from build123d import *

# Parameters (mm, degrees)
ESQUISSE1_R             = 16.5
BOSS_EXTRU_1_DEPTH      = 71
ESQUISSE2_R             = 3
BOSS_EXTRU_2_DEPTH      = 20
ESQUISSE3_W             = 2.683906319
ESQUISSE3_H             = 8.065697874
ENL_V_MAT_EXTRU_1_DEPTH = 23


with BuildPart() as part:
    # Esquisse1 → Boss.-Extru.1 (new body)
    with BuildSketch(Plane.XY):
        with Locations((-3.936360625, 11.828431373)):
            Circle(ESQUISSE1_R)
    extrude(amount=BOSS_EXTRU_1_DEPTH)

    # Esquisse2 → Boss.-Extru.2 (add)
    with BuildSketch(Plane.XY.offset(71)):
        with Locations((-3.936360625, 11.828431373)):
            Circle(ESQUISSE2_R)
    extrude(amount=BOSS_EXTRU_2_DEPTH)

    # Esquisse3 → Enlèv. mat.-Extru.1 (cut)
    with BuildSketch(Plane.XY.offset(71)):
        with Locations((-7.643790541, 11.335031517)):
            Rectangle(ESQUISSE3_W, ESQUISSE3_H)
    extrude(amount=ENL_V_MAT_EXTRU_1_DEPTH, mode=Mode.SUBTRACT)


solid = part.part
Build history of the part. All positions in model axes, mm. A direction names the side the tool comes from. Coordinates: 2 decimals unless noted, no trailing zeros. Order: outer loops, then holes, each group sorted by start corner. A loop starts at its lowest first (then second) coordinate and runs counter-clockwise, first axis right, second up. Notation, with made-up numbers: M 83.5,77 L 97.5,77 A24 cw 97.5,112 Z; hole C 6.5,-35 d11. An arc over 180 degrees is marked long. One line per question, with ' | ' between items. Start each with the question number.
Q1. Probe L1, parallel to Z at x = -15, y = 23.5; L2, parallel to Y at x = -4, z = 71.5; L3, parallel to X at y = 12.5, z = 20. List the from-to ranges inside material, lowest first. Write a range as from..to.
Q2. Saw through at D-D (y = 5). List the corners of the cut face in (x, z).
Q3. Saw through at C-C (y = 25). List the corners of the cut face in (x, z).
Q4. 3-axis set-ups, long thin cutter, end or side, ignore diameter. For faces 1 (the face through (-4, 12, 0)), 2 (the face through (-0.94, 11.72, 80.86)), 3 (the face through (-6.302, 12, 81)): which of +Z, -Z, +X, -X, +Y, -Y reach the whole face in a straight line?
Q5. Flat gauge pins, fed straight in: pin 1 Ø8 at (x, y) = (4.5, 23.5) entering from +Z; pin 2 Ø4 at (y, z) = (11.5, 80) entering from -X; pin 3 Ø4 at (x, z) = (-16, 31.5) entering from +Y. Where does each tip first touch, or does it go through?
Q6. Saw through at B-B (x = -4). List the corners of the cut face in (y, z).
Q7. Saw through at A-A (z = 79). List the corners of the cut face in (x, y), then the cut area to 3 significant figures.
Check values:
1) L1: z = 0..71 | L2: y = 8.83..14.83 | L3: x = -20.42..12.55
2) outline: M -18.96,0 L 11.08,0 L 11.08,71 L -18.96,71 Z
3) outline: M -13.87,0 L 6,0 L 6,71 L -13.87,71 Z
4) face 1: -Z, +X, -X, +Y, -Y | face 2: +Z | face 3: +Z, -X, +Y, -Y
5) pin 1: stops at z = 71 | pin 2: stops at x = -6.3 | pin 3: stops at y = 24.9
6) outline: M -4.67,0 L 28.33,0 L 28.33,71 L 14.83,71 L 14.83,91 L 8.83,91 L 8.83,71 L -4.67,71 Z
7) outline: M -6.3,9.98 A3 ccw long -6.3,13.67 Z | area: 26.7 mm2
